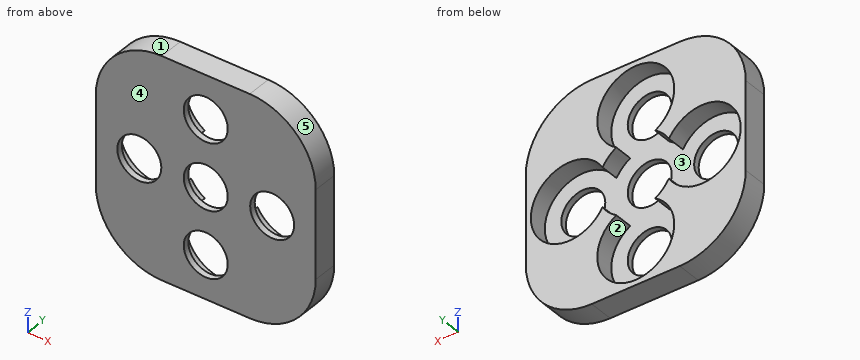
from build123d import *

# Parameters (mm, degrees)
SKETCH1_W           = 254
SKETCH1_H           = 254
BOSS_EXTRUDE1_DEPTH = 28.575
CUT_EXTRUDE1_DEPTH  = 21.59
SKETCH3_R           = 25.4
CUT_EXTRUDE2_DEPTH  = 16.51
FILLET1_R           = 76.2


with BuildPart() as part:
    # Sketch1 → Boss-Extrude1 (new body)
    with BuildSketch(Plane(origin=(0, 0, 0), x_dir=(1, 0, 0), z_dir=(0, 1, 0))):
        with Locations((127, 127)):
            Rectangle(SKETCH1_W, SKETCH1_H)
    extrude(amount=BOSS_EXTRUDE1_DEPTH)

    # Sketch2 → Cut-Extrude1 (cut)
    with BuildSketch(Plane(origin=(0, 28.575, 0), x_dir=(1, 0, 0), z_dir=(0, 1, 0))):
        with BuildLine():
            ThreePointArc((165.354, 104.532842102), (248.158, 127), (165.354, 149.467157898))
            ThreePointArc((165.354, 149.467157898), (158.430896424, 158.430896424), (149.467157898, 165.354))
            ThreePointArc((149.467157898, 165.354), (127, 248.158), (104.532842102, 165.354))
            ThreePointArc((104.532842102, 165.354), (95.569103576, 158.430896424), (88.646, 149.467157898))
            ThreePointArc((88.646, 149.467157898), (5.842, 127), (88.646, 104.532842102))
            ThreePointArc((88.646, 104.532842102), (95.569103576, 95.569103576), (104.532842102, 88.646))
            ThreePointArc((104.532842102, 88.646), (127, 5.842), (149.467157898, 88.646))
            ThreePointArc((149.467157898, 88.646), (158.430896424, 95.569103576), (165.354, 104.532842102))
        make_face()
    extrude(amount=-CUT_EXTRUDE1_DEPTH, mode=Mode.SUBTRACT)

    # Sketch3 → Cut-Extrude2 (cut)
    with BuildSketch(Plane(origin=(0, 6.985, 0), x_dir=(1, 0, 0), z_dir=(0, 1, 0))):
        with Locations(Location((127, 127, 0), (0, 0, 270))):
            Circle(SKETCH3_R)
        with Locations(Location((127, 50.292, 0), (0, 0, 270))):
            Circle(SKETCH3_R)
        with Locations(Location((50.292, 127, 0), (0, 0, 270))):
            Circle(SKETCH3_R)
        with Locations(Location((127, 203.708, 0), (0, 0, 270))):
            Circle(SKETCH3_R)
        with Locations(Location((203.708, 127, 0), (0, 0, 270))):
            Circle(SKETCH3_R)
    extrude(amount=-CUT_EXTRUDE2_DEPTH, mode=Mode.SUBTRACT)

    # Fillet1
    fillet1_edges = [part.edges().sort_by_distance(p)[0] for p in [
        (0, 14.2875, -254),
        (254, 14.2875, -254),
        (254, 14.2875, 0),
        (0, 14.2875, 0),
    ]]
    fillet(fillet1_edges, radius=FILLET1_R)


solid = part.part
Geometry check sheet. Reference: the model listing, model coordinates, mm. Face numbers are marked on the shaded views. A direction names the side the tool comes from. Round coordinates to 2 decimals unless told otherwise and drop trailing zeros. Order: outer loops, then holes, each group sorted by start corner. A loop starts at its lowest first (then second) coordinate and runs counter-clockwise, first axis right, second up. Notation, with made-up numbers: M 39.5,23.25 L 49.5,23.25 A23 ccw 49.5,35.25 Z; hole C 19,13.25 d11. An arc over 180 degrees is marked long. Write each question's results on one line, items separated by ' | '. Start each with the question number.
1. Set-up check for the marked faces 1 and 2: record each of +Z, -Z, +X, -X, +Y, -Y from which the full face is reachable in a straight line by a thin tool's end or side.
2. Draft check along X on the marked faces 3, 4 and 5. Enter one of: pulls with the +X half, pulls with the -X half, needs draft (parallel to the pull), parting line crosses it, or undercut.
3. Material ranges on L1, parallel to X at y = 1.5, z = -127; L2, parallel to Z at x = 127, y = 18.5; L3, parallel to X at y = 24.25, z = -159, recorded low to high. Write a range as from..to.
4. Cross-section at C-C on y = 17.5. Record the boundary of the cut face in (x, z).
5. Go/stop test with flat-tipped pins: P1, Ø12, axis at y = 22, z = -26.5, coming from the -X side; P2, Ø2, axis at y = 6, z = -218.5, coming from the -X side; P3, Ø2, axis at y = 15, z = -58.5, coming from the +X side. Record where each tip stops, or that it passes through.
6. Cross-section at B-B on z = -127. Record the boundary of the cut face in (x, y) (3 decimals), plus the area to 3 significant figures.
7. Cross-section at A-A on x = 127. Record the boundary of the cut face in (y, z) (3 decimals), plus the area to 3 significant figures.
8. Cross-section at D-D on x = 54. Record the boundary of the cut face in (y, z) (3 decimals), plus the area to 3 significant figures.
Resolved:
1) face 1: +Z, -X, +Y, -Y | face 2: +Y
2) face 3: undercut | face 4: needs draft | face 5: pulls with the +X half
3) L1: 0..24.89, 75.69..101.6, 152.4..178.31, 229.11..254 | L2: -254..-248.16, -5.84..0 | L3: 0..19.44, 81.14..96.15, 157.85..172.86, 234.56..254
4) outline: M 0,-177.8 A76.2 ccw 76.2,-254 L 177.8,-254 A76.2 ccw 254,-177.8 L 254,-76.2 A76.2 ccw 177.8,0 L 76.2,0 A76.2 ccw 0,-76.2 Z; hole M 88.65,-149.47 A44.45 ccw 104.53,-165.35 A44.45 ccw long 149.47,-165.35 A44.45 ccw 165.35,-149.47 A44.45 ccw long 165.35,-104.53 A44.45 ccw 149.47,-88.65 A44.45 ccw long 104.53,-88.65 A44.45 ccw 88.65,-104.53 A44.45 ccw long Z
5) P1: x = 13.78 | P2: x = 11.16 | P3: x = 252.15
6) outline: M 0,0 L 24.892,0 L 24.892,6.985 L 5.842,6.985 L 5.842,28.575 L 0,28.575 Z; M 75.692,0 L 101.6,0 L 101.6,6.985 L 75.692,6.985 Z; M 152.4,0 L 178.308,0 L 178.308,6.985 L 152.4,6.985 Z; M 229.108,0 L 254,0 L 254,28.575 L 248.158,28.575 L 248.158,6.985 L 229.108,6.985 Z | area: 962 mm2
7) outline: M 0,-254 L 28.575,-254 L 28.575,-248.158 L 6.985,-248.158 L 6.985,-229.108 L 0,-229.108 Z; M 0,-178.308 L 6.985,-178.308 L 6.985,-152.4 L 0,-152.4 Z; M 0,-101.6 L 6.985,-101.6 L 6.985,-75.692 L 0,-75.692 Z; M 0,-24.892 L 6.985,-24.892 L 6.985,-5.842 L 28.575,-5.842 L 28.575,0 L 0,0 Z | area: 962 mm2
8) outline: M 0,-250.694 L 28.575,-250.694 L 28.575,-171.295 L 6.985,-171.295 L 6.985,-152.128 L 0,-152.128 Z; M 0,-101.872 L 6.985,-101.872 L 6.985,-82.705 L 28.575,-82.705 L 28.575,-3.306 L 0,-3.306 Z | area: 4,810 mm2
